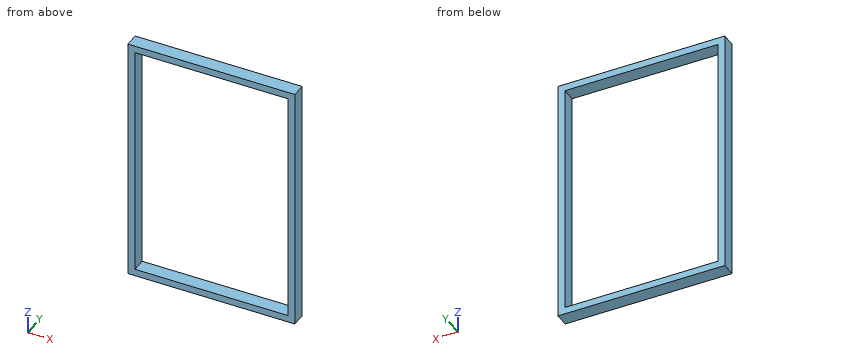
Autodesk Inventor part; units mm, degrees
ref_plane "YZ Plane" through (0, 0, 0) normal (1, 0, 0) x (0, 1, 0)
ref_plane "XZ Plane" through (0, 0, 0) normal (0, 1, 0) x (-1, 0, 0)
ref_plane "XY Plane" through (0, 0, 0) normal (0, 0, 1) x (1, 0, 0)
sketch "Sketch2" plane through (0, 0, 0) normal (0, 1, 0) x (-1, 0, 0)
  line L0 (304.8, 457.2) -> (-304.8, 457.2)
  line L1 (-304.8, 457.2) -> (-304.8, -457.2)
  line L2 (-304.8, -457.2) -> (304.8, -457.2)
  line L3 (304.8, -457.2) -> (304.8, 457.2)
  point P0 (0, 0)
  point P1 (304.8, 0)
  point P2 (0, 457.2)
  dimension "d4" = 609.6
  dimension "d5" = 914.4
extrude "Extrusion2" add sketch "Sketch2" along normal blind 50.8
sketch "Sketch3" plane through (0, 50.8, 0) normal (0, 1, 0) x (1, 0, 0)
  line L0 (279.4, -431.8) -> (279.4, 431.8)
  line L1 (279.4, 431.8) -> (-279.4, 431.8)
  line L2 (-279.4, 431.8) -> (-279.4, -431.8)
  line L3 (-279.4, -431.8) -> (279.4, -431.8)
  line L4 (279.4, -431.8) -> (-279.4, 431.8) construction
  line L5 (279.4, 431.8) -> (-279.4, -431.8) construction
  line L6 (-279.4, -431.8) -> (-304.8, -431.8)
  line L7 (-304.8, 457.2) -> (-304.8, -457.2)
  line L8 (-279.4, -431.8) -> (-279.4, -457.2)
  line L9 (279.4, -431.8) -> (279.4, -457.2)
  line L10 (-304.8, -457.2) -> (304.8, -457.2)
  line L11 (279.4, -431.8) -> (304.8, -431.8)
  line L12 (304.8, -457.2) -> (304.8, 457.2)
  line L13 (279.4, 431.8) -> (304.8, 431.8)
  line L14 (279.4, 431.8) -> (279.4, 457.2)
  line L15 (-279.4, 431.8) -> (-304.8, 431.8)
  line L16 (-279.4, 431.8) -> (-279.4, 457.2)
  line L17 (304.8, 457.2) -> (-304.8, 457.2)
  point P0 (0, 0)
  dimension "d8" = 863.6
  dimension "d9" = 558.8
extrude "Extrusion3" cut sketch "Sketch3" against normal blind 50.8 contours L3 L2 L1 L0
properties part number "Base stock holder"
Verification items for the finished model (mm, model axes). Give positions to 0.01 mm unless a question says otherwise; leave off trailing zeros. Write each loop counter-clockwise with the first axis right and the second up, starting at its lowest first coordinate (ties: lowest second). Pieces come first, ordered by that corner, then holes. Notation, with made-up numbers: (19.5, -14.75) - (61.5, -14.75) arc R27 ccw to (61.5, 19.25) - close; hole circle Ø11 at (82.25, 3). An arc over 180 degrees is marked (long way). Put each result on its own line as item: value.
Q1. Section check A-A on x = 217. Record the cut outline in (y, z).
Result:
outline: (0, -457.2) - (50.8, -457.2) - (50.8, -431.8) - (0, -431.8) - close; (0, 431.8) - (50.8, 431.8) - (50.8, 457.2) - (0, 457.2) - close
Q2. Scan lines: probe 1 along Z at (x, y) = (-114.5, 42); probe 2 along X at (y, z) = (11, 198). Record each from-to range of solid material in increasing order. Write a range as from..to.
Result:
probe 1: -457.2..-431.8, 431.8..457.2
probe 2: -304.8..-279.4, 279.4..304.8
Q3. Section check C-C on y = 40. Record the cut outline in (x, z).
Result:
outline: (-304.8, -457.2) - (304.8, -457.2) - (304.8, 457.2) - (-304.8, 457.2) - close; hole (-279.4, -431.8) - (279.4, -431.8) - (279.4, 431.8) - (-279.4, 431.8) - close
Q4. Section check B-B on z = 276.5. Record the cut outline in (x, y), and give its area (3 significant figures).
Result:
outline: (-304.8, 0) - (-279.4, 0) - (-279.4, 50.8) - (-304.8, 50.8) - close; (279.4, 0) - (304.8, 0) - (304.8, 50.8) - (279.4, 50.8) - close
area: 2,580 mm2
